Part model, mm, in its own coordinate system. A direction names the side the tool comes from. Give positions to 0.01 mm unless a question says otherwise; leave off trailing zeros. Loops run counter-clockwise (first coordinate to the right, second up) from the corner with the lowest first, then second, coordinate; pieces in that order, holes last. Notation, with made-up numbers: M 8,85.25 L 62,85.25 A26 ccw 62,105.25 Z; hole C -9.5,4.25 d7. An arc over 180 degrees is marked long. Answer in a Markdown table with one row per item.
from build123d import *

# Parameters (mm, degrees)
SKETCH_W        = 120
SKETCH_H        = 150
PAD_DEPTH       = 12
SKETCH001_R     = 50
POCKET_DEPTH    = 10
SKETCH002_R     = 47.5
POCKET001_DEPTH = 2
SKETCH003_R     = 2.65
POCKET002_DEPTH = 15
SKETCH004_R     = 1.55
POCKET003_DEPTH = 15
SKETCH005_W     = 20
SKETCH005_H     = 5
PAD001_DEPTH    = 40
SKETCH006_R     = 2.65
POCKET004_DEPTH = 5
FILLET_R        = 53
FILLET001_R     = 4
FILLET002_R     = 3
FILLET003_R     = 9.99
FILLET004_R     = 4.99


with BuildPart() as part:
    # Sketch → Pad (new body)
    with BuildSketch(Plane.XY):
        Rectangle(SKETCH_W, SKETCH_H)
    extrude(amount=PAD_DEPTH)

    # Sketch001 (on Face6 of Pad) → Pocket (cut)
    with BuildSketch(Plane.XY.offset(12)):
        with Locations((0, 15)):
            Circle(SKETCH001_R)
    extrude(amount=-POCKET_DEPTH, mode=Mode.SUBTRACT)

    # Sketch002 (on Face8 of Pocket) → Pocket001 (cut)
    with BuildSketch(Plane.XY.offset(2)):
        with Locations((0, 15)):
            Circle(SKETCH002_R)
    extrude(amount=-POCKET001_DEPTH, mode=Mode.SUBTRACT)

    # Sketch003 (on Face5 of Pocket001) → Pocket002 (cut)
    with BuildSketch(Plane.XY.offset(12)):
        with Locations((-40, -45)):
            Circle(SKETCH003_R)
        with Locations((-40, -65)):
            Circle(SKETCH003_R)
        with Locations((40, -45)):
            Circle(SKETCH003_R)
        with Locations((40, -65)):
            Circle(SKETCH003_R)
    extrude(amount=-POCKET002_DEPTH, mode=Mode.SUBTRACT)

    # Sketch004 (on Face5 of Pocket002) → Pocket003 (cut)
    with BuildSketch(Plane.XY.offset(12)):
        with Locations((-40, 55)):
            Circle(SKETCH004_R)
        with Locations((40, 55)):
            Circle(SKETCH004_R)
        with Locations((40, -25)):
            Circle(SKETCH004_R)
        with Locations((-40, -25)):
            Circle(SKETCH004_R)
    extrude(amount=-POCKET003_DEPTH, mode=Mode.SUBTRACT)

    # Sketch005 (on Face2 of Pocket003) → Pad001 (join)
    with BuildSketch(Plane.XZ.offset(75)):
        with Locations((-40, 2.5)):
            Rectangle(SKETCH005_W, SKETCH005_H)
        with Locations((40, 2.5)):
            Rectangle(SKETCH005_W, SKETCH005_H)
    extrude(amount=PAD001_DEPTH)

    # Sketch006 (on Face10 of Pad001) → Pocket004 (cut)
    with BuildSketch(Plane.XY.offset(5)):
        with Locations((-40, -105)):
            Circle(SKETCH006_R)
        with Locations((40, -105)):
            Circle(SKETCH006_R)
    extrude(amount=-POCKET004_DEPTH, mode=Mode.SUBTRACT)

    # Fillet
    fillet_edges = [part.edges().sort_by_distance(p)[0] for p in [
        (60, 75, 6),
        (-60, 75, 6),
    ]]
    fillet(fillet_edges, radius=FILLET_R)

    # Fillet001
    fillet001_edges = [part.edges().sort_by_distance(p)[0] for p in [
        (0, -75, 12),
    ]]
    fillet(fillet001_edges, radius=FILLET001_R)

    # Fillet002
    fillet002_edges = [part.edges().sort_by_distance(p)[0] for p in [
        (60, -24.5, 12),
        (-60, -24.5, 12),
    ]]
    fillet(fillet002_edges, radius=FILLET002_R)

    # Fillet003
    fillet003_edges = [part.edges().sort_by_distance(p)[0] for p in [
        (-30, -115, 2.5),
        (-50, -115, 2.5),
        (30, -115, 2.5),
        (50, -115, 2.5),
    ]]
    fillet(fillet003_edges, radius=FILLET003_R)

    # Fillet004
    fillet004_edges = [part.edges().sort_by_distance(p)[0] for p in [
        (50, -90.005, 5),
        (30, -90.005, 5),
        (-30, -90.005, 5),
        (-50, -90.005, 5),
    ]]
    fillet(fillet004_edges, radius=FILLET004_R)


solid = part.part
(1) Pull direction X, two halves, no side cores. Call faces 1 (the face through (44.06, 59.89, 4.56)), 2 (the face through (39.43, -67.59, 6.08)), 3 (the face through (-40, -92, 5)), 4 (the face through (31.423, -89.795, 3.499)): +X half, -X half, draft (parallel to the pull), parting line (faces both ways), or undercut.
Recorded:
| item | result |
|---|---|
| face 1 | +X half |
| face 2 | undercut |
| face 3 | draft |
| face 4 | undercut |
(2) Saw through at A-A (x = 0). Write the cut outline in (y, z).
Recorded:
| item | result |
|---|---|
| outline | M -75,0 L -32.5,0 L -32.5,2 L -35,2 L -35,12 L -71,12 A4 ccw -75,8 Z; M 62.5,0 L 75,0 L 75,9 A3 ccw 72,12 L 65,12 L 65,2 L 62.5,2 Z |
(3) Drill centre lines: line 1 along X through (y, z) = (13, 4); line 2 along Y through (x, z) = (-40.5, 9); line 3 along X through (y, z) = (-76.5, 0.5). Where is each one in solid material? Low to high.
Recorded:
| item | result |
|---|---|
| line 1 | x = -60 to -49.96, 49.96 to 60 |
| line 2 | y = -74.87 to -67.6, -62.4 to -47.6, -42.4 to -26.47, -23.53 to -14.32, 44.32 to 53.53, 56.47 to 63.07 |
| line 3 | x = -49.98 to -30.02, 30.02 to 49.98 |
(4) Pin check, flat tips, straight feed: pin 1 Ø5 at (x, z) = (-31.5, 5.5) entering from +Y; pin 2 Ø4 at (x, z) = (-28.5, 4.5) entering from -Y; pin 3 Ø11 at (x, y) = (41, -92.5) entering from +Z. Stop position of each tip, or through.
Recorded:
| item | result |
|---|---|
| pin 1 | stops at y = 70.22 |
| pin 2 | stops at y = -75 |
| pin 3 | stops at z = 5 |
(5) Saw through at C-C (y = -4). Write the cut outline in (x, z).
Recorded:
| item | result |
|---|---|
| outline | M -60,0 L -43.53,0 L -43.53,2 L -46.25,2 L -46.25,12 L -57,12 A3 ccw -60,9 Z; M 43.53,0 L 60,0 L 60,9 A3 ccw 57,12 L 46.25,12 L 46.25,2 L 43.53,2 Z |
(6) Which spindle directions (+Z, -Z, +X, -X, +Y, -Y) get a long thin tool onto all of the face, cutting with end or side? Do faces 5 (the face through (40, -92, 5)), 6 (the face through (48.577, -90.215, 3.499)), 7 (the face through (44.2, -3.3, 2)), 8 (the face through (-1, -75, 4)). Say none if no direction does.
Recorded:
| item | result |
|---|---|
| face 5 | +Z, +X, -X, -Y |
| face 6 | +Z, +X, -Y |
| face 7 | +Z |
| face 8 | +Z, -Y |
